```python
from build123d import *

# Parameters (mm, degrees)
SKETCH_1_R          = 17
EXTRUDE_1_DEPTH     = 15
SKETCH_2_R          = 1
CUT_EXTRUDE_1_DEPTH = 10
SKETCH_4_R          = 1.5
CUT_EXTRUDE_3_DEPTH = 2
CUT_EXTRUDE_4_REACH = 30.337
SKETCH_5_R          = 3
FILLET_1_R          = 0.5


with BuildPart() as part:
    # 草图1 → 凸台-拉伸1 (new body)
    with BuildSketch(Plane(origin=(0, 0, 0), x_dir=(1, 0, 0), z_dir=(0, 1, 0))):
        with Locations(Location((0, 0, 0), (0, 0, 270))):
            Circle(SKETCH_1_R)
    extrude(amount=EXTRUDE_1_DEPTH)

    # 草图2 → 切除-拉伸1 (cut)
    with BuildSketch(Plane(origin=(0, 15, 0), x_dir=(1, 0, 0), z_dir=(0, 1, 0))):
        with Locations(Location((0, 8, 0), (0, 0, 270))):
            Circle(SKETCH_2_R)
        with Locations(Location((0, -8, 0), (0, 0, 270))):
            Circle(SKETCH_2_R)
    extrude(amount=-CUT_EXTRUDE_1_DEPTH, mode=Mode.SUBTRACT)

    # 草图4 → 切除-拉伸3 (cut)
    with BuildSketch(Plane.XZ):
        with Locations(Location((0, 8, 0), (0, 0, 270))):
            Circle(SKETCH_4_R)
        with Locations(Location((8, 0, 0), (0, 0, 270))):
            Circle(SKETCH_4_R)
        with Locations(Location((0, -8, 0), (0, 0, 270))):
            Circle(SKETCH_4_R)
        with Locations(Location((-8, 0, 0), (0, 0, 270))):
            Circle(SKETCH_4_R)
    extrude(amount=-CUT_EXTRUDE_3_DEPTH, mode=Mode.SUBTRACT)

    # 草图5 → 切除-拉伸4 (cut, up to next)
    with BuildSketch(Plane.XZ, mode=Mode.PRIVATE) as cut_extrude_4_sk1:
        with Locations(Location((0, 0, 0), (0, 0, 270))):
            Circle(SKETCH_5_R)
    cut_extrude_4_tool1 = extrude(cut_extrude_4_sk1.sketch, amount=-CUT_EXTRUDE_4_REACH, mode=Mode.PRIVATE) & part.part
    add(cut_extrude_4_tool1.solids().sort_by_distance((0, 0, 0))[0], mode=Mode.SUBTRACT)

    # 圆角1
    fillet_1_edges = [part.edges().sort_by_distance(p)[0] for p in [
        (0, 0, -17),
        (0, 15, -17),
    ]]
    fillet(fillet_1_edges, radius=FILLET_1_R)


solid = part.part
```
The listing builds one solid part. Answer for the finished solid, in the listing's coordinates (mm). A direction names the side the tool comes from. Give positions to 0.01 mm unless a question says otherwise; leave off trailing zeros. Loops run counter-clockwise (first coordinate to the right, second up) from the corner with the lowest first, then second, coordinate; pieces in that order, holes last. Notation, with made-up numbers: (77, 42.25) - (100, 42.25) arc R8 ccw to (100, 53.25) - close; hole circle Ø2 at (45.25, 6.5). An arc over 180 degrees is marked (long way). Answer as CSV lines item,"result". Start each with the question number.
Item 1: Each of these flat-tipped pins is pushed along its axis until it touches: pin 1 (1.8 mm diameter, centred on x = -8, z = 0, fed in from -Y); pin 2 (3 mm diameter, centred on x = -11, y = 5.5, fed in from +Z); pin 3 (2 mm diameter, centred on x = 7.5, y = 10.5, fed in from -Z). Where does it stop, or does it pass through?
Item 2: The mould has two halves that part along Z. Classify faces 1 (the face through (16.855, 7.402, -2.213)), 2 (the face through (-3.4, 15, -0.2)), 3 (the face through (0, 2, -8)): +Z half, -Z half, draft (parallel to the pull), parting line (faces both ways), or undercut.
Item 3: A cutting plane is placed at D-D on y = 7. Determine the outline of the cut face in (x, z), then the cut area to 3 significant figures.
Item 4: A cutting plane is placed at B-B on x = 0. Determine the outline of the cut face in (y, z).
Item 5: Find the intervals of material crossed by line 1 (X direction, y = 0.7, z = 0); line 2 (Z direction, x = -0.5, y = 9); line 3 (X direction, y = 6.5, z = 0), in increasing order. Write a range as from..to.
Item 6: For faces 4 (the face through (6.536, 0.986, 0.325)), 5 (the face through (-1, 10, 8)), 6 (the face through (-3.4, 0, -0.2)), determine the directions among +Z, -Z, +X, -X, +Y, -Y from which every point of the face is accessible in a straight line to the end or side of a thin tool.
Item 7: A cutting plane is placed at C-C on y = 1. Determine the outline of the cut face in (x, z).
Item 8: A cutting plane is placed at A-A on z = 0. Determine the outline of the cut face in (x, y), then the cut area to 3 significant figures.
Found:
1,pin 1,"stops at y = 2"
1,pin 2,"stops at z = 14.1"
1,pin 3,"stops at z = -15.71"
2,face 1,"parting line"
2,face 2,"draft"
2,face 3,"undercut"
3,outline,"circle Ø34 at (0, 0); hole circle Ø6 at (0, 0); hole circle Ø2 at (0, -8); hole circle Ø2 at (0, 8)"
3,area,"873 mm^2"
4,outline,"(0, -16.5) arc R0.5 ccw to (0.5, -17) - (14.5, -17) arc R0.5 ccw to (15, -16.5) - (15, -9) - (5, -9) - (5, -7) - (15, -7) - (15, -3) - (0, -3) - (0, -6.5) - (2, -6.5) - (2, -9.5) - (0, -9.5) - close; (0, 3) - (15, 3) - (15, 7) - (5, 7) - (5, 9) - (15, 9) - (15, 16.5) arc R0.5 ccw to (14.5, 17) - (0.5, 17) arc R0.5 ccw to (0, 16.5) - (0, 9.5) - (2, 9.5) - (2, 6.5) - (0, 6.5) - close"
5,line 1,"x = -17..-9.5, -6.5..-3, 3..6.5, 9.5..17"
5,line 2,"z = -16.99..-8.87, -7.13..-2.96, 2.96..7.13, 8.87..16.99"
5,line 3,"x = -17..-3, 3..17"
6,face 4,"-Y"
6,face 5,"+Y"
6,face 6,"+Z, -Z, +X, -X, -Y"
7,outline,"circle Ø34 at (0, 0); hole circle Ø3 at (-8, 0); hole circle Ø6 at (0, 0); hole circle Ø3 at (0, -8); hole circle Ø3 at (0, 8); hole circle Ø3 at (8, 0)"
8,outline,"(-17, 0.5) arc R0.5 ccw to (-16.5, 0) - (-9.5, 0) - (-9.5, 2) - (-6.5, 2) - (-6.5, 0) - (-3, 0) - (-3, 15) - (-16.5, 15) arc R0.5 ccw to (-17, 14.5) - close; (3, 0) - (6.5, 0) - (6.5, 2) - (9.5, 2) - (9.5, 0) - (16.5, 0) arc R0.5 ccw to (17, 0.5) - (17, 14.5) arc R0.5 ccw to (16.5, 15) - (3, 15) - close"
8,area,"408 mm^2"
